Verification items for the finished model (mm, model axes). A direction names the side the tool comes from. Give positions to 0.01 mm unless a question says otherwise; leave off trailing zeros. Write each loop counter-clockwise with the first axis right and the second up, starting at its lowest first coordinate (ties: lowest second). Pieces come first, ordered by that corner, then holes. Notation, with made-up numbers: (-5.75, 0) -> (8.25, 0) arc R23 cw to (8.25, 12) -> close; hole circle Ø7 at (-22, 47). An arc over 180 degrees is marked (long way). Write item = value, one per line.
from build123d import *

# Parameters (mm, degrees)
SKETCH1_R           = 65
SKETCH1_R_2         = 45
BOSS_EXTRUDE1_DEPTH = 55
BOSS_EXTRUDE2_DEPTH = 30


with BuildPart() as part:
    # Sketch1 → Boss-Extrude1 (new body)
    with BuildSketch(Plane.XY):
        Circle(SKETCH1_R)
        Circle(SKETCH1_R_2, mode=Mode.SUBTRACT)
    extrude(amount=BOSS_EXTRUDE1_DEPTH)

    # Sketch2 → Boss-Extrude2 (add)
    with BuildSketch(Plane(origin=(0, 0, 0), x_dir=(-1, 0, 0), z_dir=(0, 0, -1))):
        with BuildLine():
            Line((-5, -75), (5, -75))
            ThreePointArc((5, -75), (54.497474683, -54.497474683), (75, -5))
            Line((75, -5), (75, 5))
            ThreePointArc((75, 5), (54.497474683, 54.497474683), (5, 75))
            Line((5, 75), (-5, 75))
            ThreePointArc((-5, 75), (-54.497474683, 54.497474683), (-75, 5))
            Line((-75, 5), (-75, -5))
            ThreePointArc((-75, -5), (-54.497474683, -54.497474683), (-5, -75))
        make_face()
    extrude(amount=BOSS_EXTRUDE2_DEPTH)


solid = part.part
Item 1: Set-up check for faces 4 (the cylindrical face through (20.765, -39.923, 27.115)), 5 (the cylindrical face through (-53.95, -55.04, -14.79)): record each of +Z, -Z, +X, -X, +Y, -Y from which the full face is reachable in a straight line by a thin tool's end or side.
Response values:
face_4 = +Z
face_5 = +Z, -Z, -X, -Y
Item 2: Sectioned sample at D-D on z = 18. Record the cut outline in (x, y), then the cut area to 3 significant figures.
Response values:
outline = circle Ø130 at (0, 0); hole circle Ø90 at (0, 0)
area = 6,910 mm^2
Item 3: Material ranges on line 1 (Y direction, x = 0, z = 30.5); line 2 (Z direction, x = 22.5, y = 67); line 3 (X direction, y = -22, z = 45.5), recorded low to high.
Response values:
line_1 = -65 to -45, 45 to 65
line_2 = -30 to 0
line_3 = -61.16 to -39.26, 39.26 to 61.16
Item 4: Sectioned sample at B-B on z = -7. Record the cut outline in (x, y).
Response values:
outline = (-75, -5) arc R70 ccw to (-5, -75) -> (5, -75) arc R70 ccw to (75, -5) -> (75, 5) arc R70 ccw to (5, 75) -> (-5, 75) arc R70 ccw to (-75, 5) -> close
Item 5: Sectioned sample at A-A on y = 0. Record the cut outline in (x, z), then the cut area to 3 significant figures.
Response values:
outline = (-75, -30) -> (75, -30) -> (75, 0) -> (65, 0) -> (65, 55) -> (45, 55) -> (45, 0) -> (-45, 0) -> (-45, 55) -> (-65, 55) -> (-65, 0) -> (-75, 0) -> close
area = 6,700 mm^2
Item 6: Mould release check, pull along Y, two halves, no side actions. Record for faces 1 (the flat face through (1, 1, 0)), 2 (the flat face through (0, 75, -15)), 3 (the cylindrical face through (55.04, -53.95, -14.79)): +Y half, -Y half, draft (parallel to the pull), parting line (faces both ways), or undercut.
Response values:
face_1 = undercut
face_2 = +Y half
face_3 = -Y half
Item 7: Go/stop test with flat-tipped pins: P1, Ø12, axis at x = 44, z = -8.5, coming from the -Y side; P2, Ø8, axis at x = -13, z = 20, coming from the -Y side; P3, Ø1.5, axis at x = 58.5, z = -13.5, coming from the +Y side. Record where each tip stops, or that it passes through.
Response values:
P1 = -66.73
P2 = -64.37
P3 = 51.02
